The model under review builds one solid part; all positions refer to its coordinate system, in mm. Face numbers are marked on the shaded views. Round coordinates to 2 decimals unless told otherwise and drop trailing zeros. Order: outer loops, then holes, each group sorted by start corner. A loop starts at its lowest first (then second) coordinate and runs counter-clockwise, first axis right, second up.
```python
from build123d import *

# Parameters (mm, degrees)
SKETCH1_W            = 35.56
SKETCH1_H            = 15.9512
BOSS_EXTRUDE1_DEPTH  = 1.397
SKETCH14_W           = 27.0002
SKETCH14_H           = 12.827
BOSS_EXTRUDE14_DEPTH = 1.016
SKETCH15_W           = 4.572
SKETCH15_H           = 11.43
BOSS_EXTRUDE15_DEPTH = 0.1016
SKETCH16_W           = 0.1016
SKETCH16_H           = 10.795
CUT_EXTRUDE1_DEPTH   = 3.937
SKETCH17_W           = 2.54
SKETCH17_H           = 9.525
BOSS_EXTRUDE16_DEPTH = 0.1016
SKETCH18_W           = 2.54
SKETCH18_H           = 3.175
CUT_EXTRUDE2_DEPTH   = 0.1016
SKETCH19_W           = 2.54
SKETCH19_H           = 1.905
BOSS_EXTRUDE17_DEPTH = 0.1016
SKETCH20_W           = 2.54
SKETCH20_H           = 0.635
CUT_EXTRUDE3_DEPTH   = 0.1016
SKETCH21_W           = 2.54
SKETCH21_H           = 0.635
CUT_EXTRUDE4_DEPTH   = 0.1016
SKETCH22_W           = 2.54
SKETCH22_H           = 3.175
CUT_EXTRUDE5_DEPTH   = 0.1016
SKETCH23_W           = 2.54
SKETCH23_H           = 1.905
BOSS_EXTRUDE18_DEPTH = 0.1016
SKETCH24_W           = 2.54
SKETCH24_H           = 0.635
CUT_EXTRUDE6_DEPTH   = 0.1016
SKETCH25_W           = 1.3462
SKETCH25_H           = 0.381
BOSS_EXTRUDE19_DEPTH = 0.762
SKETCH26_W           = 6.35
SKETCH26_H           = 8.382
BOSS_EXTRUDE20_DEPTH = 0.8382
SKETCH27_W           = 8.382
SKETCH27_H           = 8.382
BOSS_EXTRUDE21_DEPTH = 0.8382
SKETCH28_W           = 2.54
SKETCH28_H           = 2.032
BOSS_EXTRUDE22_DEPTH = 0.508
HOLE1_D              = 0.7366
HOLE1_DEPTH          = 3.2512


with BuildPart() as part:
    # Sketch1 → Boss-Extrude1 (new body)
    with BuildSketch(Plane(origin=(-73.738355388, 0, 0), x_dir=(0, 0, -1), z_dir=(1, 0, 0))):
        with Locations((-23.5966, 48.047439016)):
            Rectangle(SKETCH1_W, SKETCH1_H)
    extrude(amount=-BOSS_EXTRUDE1_DEPTH)

    # Sketch14 → Boss-Extrude14 (add)
    with BuildSketch(Plane(origin=(-73.738355388, 0, 0), x_dir=(0, 0, -1), z_dir=(1, 0, 0))):
        with Locations((-27.1145, 48.047439016)):
            Rectangle(SKETCH14_W, SKETCH14_H)
    extrude(amount=BOSS_EXTRUDE14_DEPTH)

    # Sketch15 → Boss-Extrude15 (add)
    with BuildSketch(Plane(origin=(-72.722355388, 0, 0), x_dir=(0, 0, -1), z_dir=(1, 0, 0))):
        with Locations((-38.227, 47.348939016)):
            Rectangle(SKETCH15_W, SKETCH15_H)
    extrude(amount=BOSS_EXTRUDE15_DEPTH)

    # Sketch16 → Cut-Extrude1 (cut)
    with BuildSketch(Plane(origin=(0, 0, 35.941), x_dir=(-1, 0, 0), z_dir=(0, 0, -1))):
        with Locations((72.671555388, 47.031439016)):
            Rectangle(SKETCH16_W, SKETCH16_H)
    extrude(amount=-CUT_EXTRUDE1_DEPTH, mode=Mode.SUBTRACT)

    # Sketch17 → Boss-Extrude16 (add)
    with BuildSketch(Plane(origin=(-72.722355388, 0, 0), x_dir=(0, 0, -1), z_dir=(1, 0, 0))):
        with Locations((-38.608, 47.031439016)):
            Rectangle(SKETCH17_W, SKETCH17_H)
    extrude(amount=BOSS_EXTRUDE16_DEPTH)

    # Sketch18 → Cut-Extrude2 (cut)
    with BuildSketch(Plane(origin=(-72.620755388, 0, 0), x_dir=(0, 0, -1), z_dir=(1, 0, 0))):
        with Locations((-39.243, 49.571439016)):
            Rectangle(SKETCH18_W, SKETCH18_H)
    extrude(amount=-CUT_EXTRUDE2_DEPTH, mode=Mode.SUBTRACT)

    # Sketch19 → Boss-Extrude17 (add)
    with BuildSketch(Plane(origin=(-72.722355388, 0, 0), x_dir=(0, 0, -1), z_dir=(1, 0, 0))):
        with Locations((-39.243, 49.571439016)):
            Rectangle(SKETCH19_W, SKETCH19_H)
    extrude(amount=BOSS_EXTRUDE17_DEPTH)

    # Sketch20 → Cut-Extrude3 (cut)
    with BuildSketch(Plane(origin=(-72.620755388, 0, 0), x_dir=(0, 0, -1), z_dir=(1, 0, 0))):
        with Locations((-38.608, 49.571439016)):
            Rectangle(SKETCH20_W, SKETCH20_H)
    extrude(amount=-CUT_EXTRUDE3_DEPTH, mode=Mode.SUBTRACT)

    # Sketch21 → Cut-Extrude4 (cut)
    with BuildSketch(Plane(origin=(-72.620755388, 0, 0), x_dir=(0, 0, -1), z_dir=(1, 0, 0))):
        with Locations((-38.608, 47.031439016)):
            Rectangle(SKETCH21_W, SKETCH21_H)
    extrude(amount=-CUT_EXTRUDE4_DEPTH, mode=Mode.SUBTRACT)

    # Sketch22 → Cut-Extrude5 (cut)
    with BuildSketch(Plane(origin=(-72.620755388, 0, 0), x_dir=(0, 0, -1), z_dir=(1, 0, 0))):
        with Locations((-39.243, 44.491439016)):
            Rectangle(SKETCH22_W, SKETCH22_H)
    extrude(amount=-CUT_EXTRUDE5_DEPTH, mode=Mode.SUBTRACT)

    # Sketch23 → Boss-Extrude18 (add)
    with BuildSketch(Plane(origin=(-72.722355388, 0, 0), x_dir=(0, 0, -1), z_dir=(1, 0, 0))):
        with Locations((-39.243, 44.491439016)):
            Rectangle(SKETCH23_W, SKETCH23_H)
    extrude(amount=BOSS_EXTRUDE18_DEPTH)

    # Sketch24 → Cut-Extrude6 (cut)
    with BuildSketch(Plane(origin=(-72.620755388, 0, 0), x_dir=(0, 0, -1), z_dir=(1, 0, 0))):
        with Locations((-38.608, 44.491439016)):
            Rectangle(SKETCH24_W, SKETCH24_H)
    extrude(amount=-CUT_EXTRUDE6_DEPTH, mode=Mode.SUBTRACT)

    # Sketch25 → Boss-Extrude19 (add)
    with BuildSketch(Plane(origin=(-72.722355388, 0, 0), x_dir=(0, 0, -1), z_dir=(1, 0, 0))):
        with Locations((-23.0505, 44.288239016)):
            Rectangle(SKETCH25_W, SKETCH25_H)
    extrude(amount=BOSS_EXTRUDE19_DEPTH)

    # Sketch26 → Boss-Extrude20 (add)
    with BuildSketch(Plane(origin=(-72.722355388, 0, 0), x_dir=(0, 0, -1), z_dir=(1, 0, 0))):
        with Locations((-18.0594, 49.660339016)):
            Rectangle(SKETCH26_W, SKETCH26_H)
    extrude(amount=BOSS_EXTRUDE20_DEPTH)

    # Sketch27 → Boss-Extrude21 (add)
    with BuildSketch(Plane(origin=(-72.722355388, 0, 0), x_dir=(0, 0, -1), z_dir=(1, 0, 0))):
        with Locations((-26.9494, 49.660339016)):
            Rectangle(SKETCH27_W, SKETCH27_H)
    extrude(amount=BOSS_EXTRUDE21_DEPTH)

    # Sketch28 → Boss-Extrude22 (add)
    with BuildSketch(Plane(origin=(-72.722355388, 0, 0), x_dir=(0, 0, -1), z_dir=(1, 0, 0))):
        with Locations((-29.8704, 43.945339016)):
            Rectangle(SKETCH28_W, SKETCH28_H)
    extrude(amount=BOSS_EXTRUDE22_DEPTH)

    # Hole1
    with Locations(Plane.ZY.offset(75.135355388)):
        with Locations((7.3025, 41.557739016), (7.3025, 54.537139016)):
            Hole(HOLE1_D / 2, depth=HOLE1_DEPTH)


solid = part.part
```
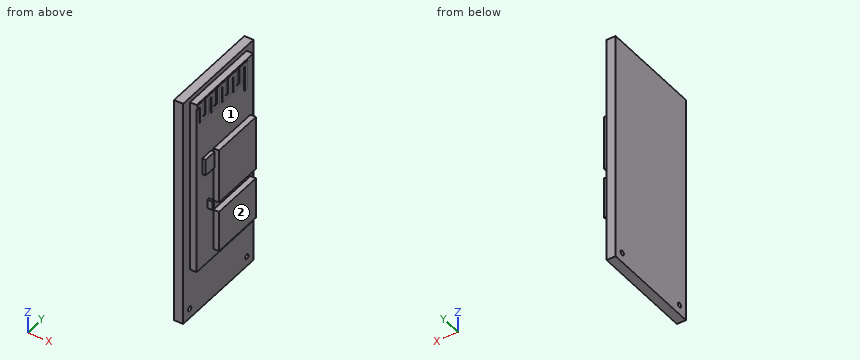
(1) Consider section A-A (z = 32). Write out the cut boundary in (x, y).
Data:
outline: (-75.14, 40.07) - (-73.74, 40.07) - (-73.74, 41.63) - (-72.72, 41.63) - (-72.72, 54.46) - (-73.74, 54.46) - (-73.74, 56.02) - (-75.14, 56.02) - close
(2) Consider section C-C (z = 13). Write out the cut boundary in (x, y).
Data:
outline: (-75.14, 40.07) - (-73.74, 40.07) - (-73.74, 56.02) - (-75.14, 56.02) - close
(3) To check wall thickness, follow probe 1 along Z at (x, y) = (-72.35, 47.75); probe 2 along Y at (x, z) = (-72.5, 28); probe 3 along Z at (x, y) = (-73.2, 52.5). State the ranges of each line that lie inside material, in increasing order.
Data:
probe 1: z = 14.88 to 21.23, 22.76 to 31.14
probe 2: y = 45.47 to 53.85
probe 3: z = 13.61 to 40.61
(4) Draft analysis for pull direction Z (two halves, no side actions). For the marked faces 1 and 2, state which applies: pulls with the +Z half, pulls with the -Z half, needs draft (parallel to the pull), parting line crosses it, or undercut.
Data:
face 1: undercut
face 2: needs draft
(5) Insertion check: pin 1 (1.5 mm diameter, centred on x = -72.5, y = 43, fed in from -Z); pin 2 (0.9 mm diameter, centred on x = -72.5, z = 25, fed in from +Y); pin 3 (0.6 mm diameter, centred on x = -72.5, z = 22.5, fed in from -Y). Each pin has a flat end and moves straight along its axis. Give the tip position at first contact, or say it passes through.
Data:
pin 1: stops at z = 13.61
pin 2: stops at y = 54.46
pin 3: stops at y = 41.63
(6) Consider section B-B (x = -73.1). Write out the cut boundary in (y, z).
Data:
outline: (41.63, 13.61) - (54.46, 13.61) - (54.46, 40.61) - (41.63, 40.61) - close
